from build123d import *

# Parameters (mm, degrees)
SKETCH1_W      = 125
SKETCH1_H      = 125
SKETCH1_R      = 1.4
EXTRUDE1_DEPTH = 1.5
EXTRUDE2_DEPTH = 10


with BuildPart() as part:
    # Sketch1 → Extrude1 (new body)
    with BuildSketch(Plane.XY):
        Rectangle(SKETCH1_W, SKETCH1_H)
        with Locations((46.0375, 38.1)):
            Circle(SKETCH1_R, mode=Mode.SUBTRACT)
        with Locations((38.1, 46.0375)):
            Circle(SKETCH1_R, mode=Mode.SUBTRACT)
        with Locations((-38.1, 46.0375)):
            Circle(SKETCH1_R, mode=Mode.SUBTRACT)
        with Locations((-46.0375, 38.1)):
            Circle(SKETCH1_R, mode=Mode.SUBTRACT)
        with Locations((-46.0375, -38.1)):
            Circle(SKETCH1_R, mode=Mode.SUBTRACT)
        with Locations((-38.1, -46.0375)):
            Circle(SKETCH1_R, mode=Mode.SUBTRACT)
        with Locations((38.1, -46.0375)):
            Circle(SKETCH1_R, mode=Mode.SUBTRACT)
        with Locations((46.0375, -38.1)):
            Circle(SKETCH1_R, mode=Mode.SUBTRACT)
    extrude(amount=EXTRUDE1_DEPTH)

    # Sketch2 → Extrude2 (cut)
    with BuildSketch(Plane.XY.offset(1.5)):
        Polygon((41.063122539, -62.5), (62.5, -44.338577872), (62.5, -62.5), align=None)
        Polygon((41.063122539, 62.5), (62.5, 41.063122539), (62.5, 62.5), align=None)
        Polygon((-41.384179801, -62.5), (-62.5, -41.384179801), (-62.5, -62.5), align=None)
        Polygon((-62.5, 41.063122539), (-41.063122539, 62.5), (-62.5, 62.5), align=None)
    extrude(amount=-EXTRUDE2_DEPTH, mode=Mode.SUBTRACT)


solid = part.part
Source: CAD feature listing. Evaluate the final solid. Frame: model axes, mm. Round coordinates to 2 decimals unless told otherwise and drop trailing zeros. Loops run counter-clockwise (first coordinate to the right, second up) from the corner with the lowest first, then second, coordinate; pieces in that order, holes last. Notation, with made-up numbers: M 3,-37.75 L 12,-37.75 A36 cw 12,1.25 Z; hole C 59.5,72.5 d8. An arc over 180 degrees is marked long. Return JSON: item names as keys, results as strings. Group by question number.
1. Section query A-A on z = 0.55. State how many separate pieces and enclosed holes the cut face has, and give its area (3 significant figures).
2. Pin query (flat end, axial travel): pin 1 (2.5 mm diameter, centred on x = -46.04, y = -38.1, fed in from -Z). Return the tip coordinate at first contact, or that it passes through.
3. Section query C-C on x = -54. Output: boundary loops of the cut face in (y, z).
4. Section query B-B on x = 53. Output: boundary loops of the cut face in (y, z), and give its area (3 significant figures).
5. Mould query, pull axis X, two halves, no side actions, for faces 1 (the face through (-1, 1, 0)), 2 (the face through (-51.932, 51.632, 0.76)), 3 (the face through (-38.282, 47.426, 0.74)). Classes: released by +X, released by -X, zero draft, split by the parting line, or undercut.
6. Material intervals for line 1 along Y through (x, z) = (-38, 1.15); line 2 along Y through (x, z) = (-37, 0.2); line 3 along Y through (x, z) = (-52, 1.25), sorted ascending. Write a range as from..to.
Checks:
{
 "1": {"separate pieces": "1", "enclosed holes": "8", "area": "14,700 mm²"},
 "2": {"pin 1": "passes through"},
 "3": {"outline": "M -49.88,0 L 49.56,0 L 49.56,1.5 L -49.88,1.5 Z"},
 "4": {"outline": "M -52.39,0 L 50.56,0 L 50.56,1.5 L -52.39,1.5 Z", "area": "154 mm²"},
 "5": {"face 1": "zero draft", "face 2": "released by -X", "face 3": "undercut"},
 "6": {"line 1": "y = -62.5..-47.43, -44.64..44.64, 47.43..62.5", "line 2": "y = -62.5..-46.9, -45.17..45.17, 46.9..62.5", "line 3": "y = -51.88..51.56"}
}
